Read the model definition and answer for the solid it produces. Units are mm, in the model's axes. A direction names the side the tool comes from. Give positions to 0.01 mm unless a question says otherwise; leave off trailing zeros. Order: outer loops, then holes, each group sorted by start corner. A loop starts at its lowest first (then second) coordinate and runs counter-clockwise, first axis right, second up.
Item 1: Which of the six approach directions +Z, -Z, +X, -X, +Y, -Y give full straight-line access (tool end or side, diameter ignored) to faces 5 (the face through (3, -30, 59)), 6 (the face through (3, 0, -40)), 7 (the face through (2.84, -12.86, -27.73)), 8 (the face through (3, 15, 59))?
Item 2: A cutting plane is placed at D-D (x = 2.7). State how many separate pieces and enclosed holes the cut face has, plus the area to 3 significant figures.
Item 3: Find the intervals of material crossed by line 1 along Y through (x, z) = (1.75, 62.8); line 2 along Y through (x, z) = (1.15, -44); line 3 along Y through (x, z) = (2.85, -62.8), in increasing order.
Item 4: A cutting plane is placed at A-A (z = -62.8). Write down the section's boundary in (x, y), plus the area to 3 significant figures.
Item 5: A cutting plane is placed at B-B (y = 25). Write down the section's boundary in (x, z).
Item 6: Given pin 1 Ø1.7 at (x, z) = (3.5, 57) entering from -Y; pin 2 Ø3 at (x, y) = (1.5, 11.5) entering from -Z; pin 3 Ø1.7 at (x, z) = (3, -56) entering from +Y; pin 4 Ø2.5 at (y, z) = (-20, 62.8) entering from -X (1 decimal), each flat-ended and moving along its own axis, determine where each tip first touches the part or whether it passes through.
Item 7: A cutting plane is placed at C-C (z = 62.8). Write down the section's boundary in (x, y), plus the area to 3 significant figures.
Item 8: The mould has two halves that part along Y. Classify faces 1 (the face through (2.839, -25.707, 15.631)), 2 (the face through (3, 25, 67.8)), 3 (the face through (3, -30, -59)), 4 (the face through (2.76, 25.07, 64.4)): +Y half, -Y half, draft (parallel to the pull), parting line (faces both ways), or undercut.
from build123d import *

# Parameters (mm, degrees)
SKETCH_1_W          = 104
SKETCH_1_H          = 80
SKETCH_1_W_2        = 15.8
SKETCH_1_H_2        = 20
SKETCH_1_R          = 1.6
EXTRUDE_1_DEPTH     = 5.6
FILLET_1_R          = 5
CUT_EXTRUDE_1_DEPTH = 79.918945761
SKETCH_4_W          = 12
SKETCH_4_H          = 12
CUT_EXTRUDE_2_DEPTH = 79.918945761
FILLET_2_R          = 2


with BuildPart() as part:
    # ｽｹｯﾁ1 → ﾎﾞｽ - 押し出し1 (new body)
    # profile 1 of 4: a face of its own
    with BuildSketch(Plane(origin=(0, 0, 0), x_dir=(0, 0, -1), z_dir=(1, 0, 0))):
        Rectangle(SKETCH_1_W, SKETCH_1_H)
    # profile 2 of 4: a face of its own
    with BuildSketch(Plane(origin=(0, 0, 0), x_dir=(0, 0, -1), z_dir=(1, 0, 0))):
        with Locations((-59.9, 25)):
            Rectangle(SKETCH_1_W_2, SKETCH_1_H_2)
        with Locations((-62.8, 25)):
            Circle(SKETCH_1_R, mode=Mode.SUBTRACT)
    # profile 3 of 4: a face of its own
    with BuildSketch(Plane(origin=(0, 0, 0), x_dir=(0, 0, -1), z_dir=(1, 0, 0))):
        with Locations((59.9, -20)):
            Rectangle(SKETCH_1_W_2, SKETCH_1_H_2)
        with Locations((62.8, -20)):
            Circle(SKETCH_1_R, mode=Mode.SUBTRACT)
    # profile 4 of 4: a face of its own
    with BuildSketch(Plane(origin=(0, 0, 0), x_dir=(0, 0, -1), z_dir=(1, 0, 0))):
        with Locations((-59.9, -20)):
            Rectangle(SKETCH_1_W_2, SKETCH_1_H_2)
        with Locations((-62.8, -20)):
            Circle(SKETCH_1_R, mode=Mode.SUBTRACT)
    extrude(amount=EXTRUDE_1_DEPTH)

    # ﾌｨﾚｯﾄ1
    fillet_1_edges = [part.edges().sort_by_distance(p)[0] for p in [
        (2.8, -40, -52),
        (2.8, -40, 52),
        (2.8, 40, 52),
        (2.8, 40, -52),
    ]]
    fillet(fillet_1_edges, radius=FILLET_1_R - 0.0001)  # a hair under: the kernel refuses the full size

    # ｽｹｯﾁ3 → ｶｯﾄ - 押し出し1 (cut, through all)
    with BuildSketch(Plane(origin=(5.6, 0, 0), x_dir=(0, 0, -1), z_dir=(1, 0, 0))):
        Polygon((-24.896207629, -29.079798567), (-6.102355213, -22.2393957), (-4.187042411, -27.501674377), (-22.980894827, -34.342077243), align=None)
        Polygon((7.993034098, -17.10909355), (26.786886514, -10.268690684), (28.702199317, -15.53096936), (9.908346901, -22.371372227), align=None)
    extrude(amount=-CUT_EXTRUDE_1_DEPTH, mode=Mode.SUBTRACT)

    # ｽｹｯﾁ4 → ｶｯﾄ - 押し出し2 (cut, through all)
    with BuildSketch(Plane(origin=(5.6, 0, 0), x_dir=(0, 0, -1), z_dir=(1, 0, 0))):
        with Locations((-46, 0)):
            Rectangle(SKETCH_4_W, SKETCH_4_H)
        with Locations((46, 0)):
            Rectangle(SKETCH_4_W, SKETCH_4_H)
    extrude(amount=-CUT_EXTRUDE_2_DEPTH, mode=Mode.SUBTRACT)

    # ﾌｨﾚｯﾄ2
    fillet_2_edges = [part.edges().sort_by_distance(p)[0] for p in [
        (2.8, -6, 52),
        (2.8, 6, 52),
        (2.8, 6, -52),
        (2.8, -6, -52),
        (2.8, -10, -67.8),
        (2.8, -30, -67.8),
        (2.8, -30, 67.8),
        (2.8, -10, 67.8),
        (2.8, 15, 67.8),
        (2.8, 35, 67.8),
    ]]
    fillet(fillet_2_edges, radius=FILLET_2_R)


solid = part.part
Response values:
1. face 5: +Z, +X, -X, -Y
1. face 6: -Z, +X, -X
1. face 7: +X, -X
1. face 8: +Z, +X, -X
2. separate pieces: 1
2. enclosed holes: 5
2. area: 8,700 mm2
3. line 1: y = -30 to -21.6, -18.4 to -10, 15 to 23.4, 26.6 to 35
3. line 2: y = -40 to -6, 6 to 40
3. line 3: y = -30 to -21.6, -18.4 to -10
4. outline: (0, -30) - (5.6, -30) - (5.6, -21.6) - (0, -21.6) - close; (0, -18.4) - (5.6, -18.4) - (5.6, -10) - (0, -10) - close
4. area: 94.1 mm2
5. outline: (0, -52) - (5.6, -52) - (5.6, 61.2) - (0, 61.2) - close; (0, 64.4) - (5.6, 64.4) - (5.6, 67.8) - (0, 67.8) - close
6. pin 1: stops at y = -30
6. pin 2: stops at z = -52
6. pin 3: stops at y = -10
6. pin 4: passes through
7. outline: (0, -30) - (5.6, -30) - (5.6, -21.6) - (0, -21.6) - close; (0, -18.4) - (5.6, -18.4) - (5.6, -10) - (0, -10) - close; (0, 15) - (5.6, 15) - (5.6, 23.4) - (0, 23.4) - close; (0, 26.6) - (5.6, 26.6) - (5.6, 35) - (0, 35) - close
7. area: 188 mm2
8. face 1: undercut
8. face 2: draft
8. face 3: -Y half
8. face 4: undercut
